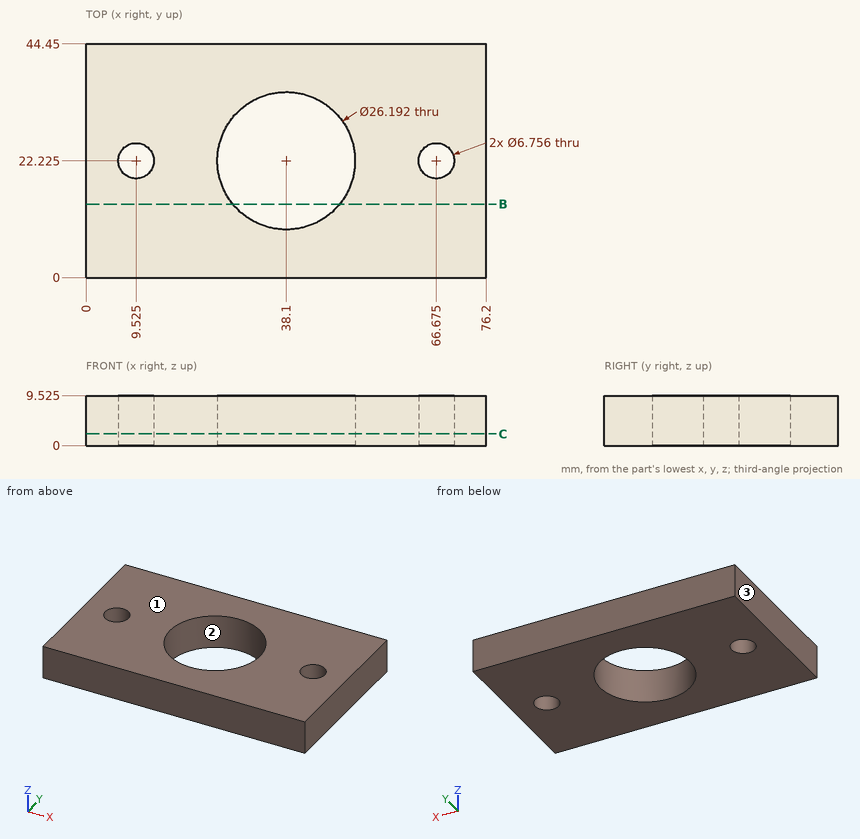
Geometry check sheet. Reference: drawing and pictorial views, mm from the part's lowest x, y, z. Round coordinates to 2 decimals unless told otherwise and drop trailing zeros. Order: outer loops, then holes, each group sorted by start corner. A loop starts at its lowest first (then second) coordinate and runs counter-clockwise, first axis right, second up. Notation, with made-up numbers: (29.5, -4) - (50.5, -4) arc R22 ccw to (50.5, 8) - close; hole circle Ø8 at (84.5, 63.25). An arc over 180 degrees is marked (long way). Use a Markdown table: item, result. Add a question column.
1) Section check B-B (y = 14). Record the cut outline in (x, z) (1 decimal), then the cut area to 3 significant figures.
2) Thickness scan on line 1 along Y through (x, z) = (66.5, 7); line 2 along X through (y, z) = (12.5, 3); line 3 along X through (y, z) = (29.5, 4.75). Record the ranges inside material, lowest first.
3) Section check C-C (z = 2.25). Count the separate pieces of the cut face and the enclosed holes in it, then the cut area to 3 significant figures.
4) Mould release check, pull along X, two halves, no side actions. Record for the marked faces 1, 2 and 3: released by +X, released by -X, zero draft, split by the parting line, or undercut.
Established:
| question | item | result |
|---|---|---|
| 1 | outline | (0, 0) - (27.9, 0) - (27.9, 9.5) - (0, 9.5) - close; (48.3, 0) - (76.2, 0) - (76.2, 9.5) - (48.3, 9.5) - close |
| 1 | area | 532 mm2 |
| 2 | line 1 | 0 to 18.85, 25.6 to 44.45 |
| 2 | line 2 | 0 to 29.33, 46.87 to 76.2 |
| 2 | line 3 | 0 to 27.21, 48.99 to 76.2 |
| 3 | separate pieces | 1 |
| 3 | enclosed holes | 3 |
| 3 | area | 2,780 mm2 |
| 4 | face 1 | zero draft |
| 4 | face 2 | undercut |
| 4 | face 3 | released by -X |
